Verification items for the finished model (mm, model axes). Face numbers are marked on the shaded views. Round coordinates to 2 decimals unless told otherwise and drop trailing zeros. Order: outer loops, then holes, each group sorted by start corner. A loop starts at its lowest first (then second) coordinate and runs counter-clockwise, first axis right, second up. Notation, with made-up numbers: (-21.75, 80) -> (19.25, 80) arc R29 ccw to (19.25, 116) -> close; hole circle Ø5 at (-14, 15). An arc over 180 degrees is marked (long way). Return JSON: item names as keys, results as strings. Group by question number.
Item 1: Scan lines: probe 1 along Z at (x, y) = (-12, 18.5); probe 2 along X at (y, z) = (26.5, 0); probe 3 along Z at (x, y) = (6, 37). Record each from-to range of solid material in increasing order. Write a range as from..to.
Item 2: Sectioned sample at D-D on x = 15. Record the cut outline in (y, z).
Item 3: Sectioned sample at C-C on z = 0. Record the cut outline in (x, y), plus the area to 3 significant figures.
Item 4: Draft check along X on the marked faces 1, 2 and 3. Enter one of: pulls with the +X half, pulls with the -X half, needs draft (parallel to the pull), parting line crosses it, or undercut.
Item 5: Sectioned sample at B-B on y = 18.5. Record the cut outline in (x, z).
Item 6: Sectioned sample at A-A on x = -14. Record the cut outline in (y, z), plus the area to 3 significant figures.
Autodesk Inventor part; units mm, degrees
ref_plane "YZ Plane" through (0, 0, 0) normal (1, 0, 0) x (0, 1, 0)
ref_plane "XZ Plane" through (0, 0, 0) normal (0, 1, 0) x (-1, 0, 0)
ref_plane "XY Plane" through (0, 0, 0) normal (0, 0, 1) x (1, 0, 0)
sketch "스케치1" plane through (0, 0, 0) normal (0, 1, 0) x (-1, 0, 0)
  line L0 (0, -16.483) -> (0, 16.483)
  line L1 (31.8385, 0) -> (-30.0309, 0)
  arc A0 (16.9497, 4.9497) -> (16.9497, -4.9497) centre (12, 0) ccw
  line L2 (12, -11) -> (0, -11)
  line L3 (12, 11) -> (0, 11)
  line L4 (12, 0) -> (19.7782, -7.7782)
  line L5 (12, 0) -> (23, 0) construction
  arc A1 (19.7782, -7.7782) -> (16.9497, -4.9497) centre (18.364, -6.364) ccw
  arc A2 (16.9497, 4.9497) -> (19.7782, 7.7782) centre (18.364, 6.364) ccw
  arc A3 (12, -11) -> (19.7782, -7.7782) centre (12, 0) ccw
  arc A4 (19.7782, 7.7782) -> (12, 11) centre (12, 0) ccw
  arc A5 (-16.9497, -4.9497) -> (-16.9497, 4.9497) centre (-12, 0) ccw
  line L6 (-12, -11) -> (0, -11)
  arc A6 (-16.9497, -4.9497) -> (-19.7782, -7.7782) centre (-18.364, -6.364) ccw
  arc A7 (-19.7782, 7.7782) -> (-16.9497, 4.9497) centre (-18.364, 6.364) ccw
  arc A8 (-19.7782, -7.7782) -> (-12, -11) centre (-12, 0) ccw
  arc A9 (-12, 11) -> (-19.7782, 7.7782) centre (-12, 0) ccw
  line L7 (-12, 11) -> (0, 11)
  point P0 (0, 0)
  dimension "d0" = 14
  dimension "d1" = 12
  dimension "d3" = 45
  dimension "d4" = 11
extrude "돌출1" add sketch "스케치1" along normal blind 50 contours L6 A8 A6 A5 L1 L0 | L0 L1 A0 L4 A3 L2 | L1 A5 A7 A9 L7 L0 | L0 L3 A4 A2 A0 L1 | L4 A1
properties part number "카메라 고정 중단"
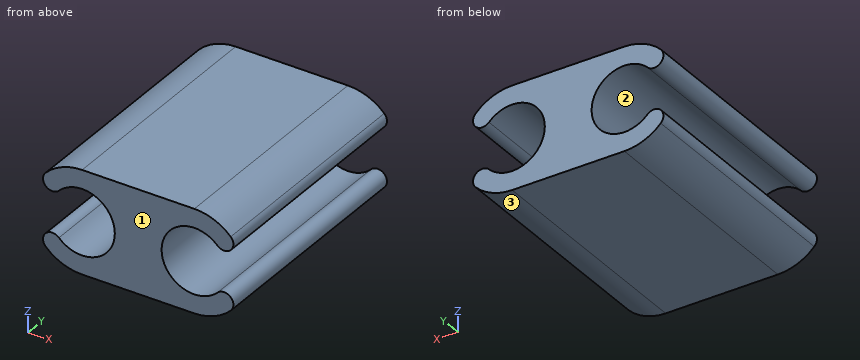
Recorded:
{
 "1": {"probe 1": "-11..-7, 7..11", "probe 2": "-5..5", "probe 3": "-11..-3.61, 3.61..11"},
 "2": {"outline": "(0, -10.58) -> (50, -10.58) -> (50, -6.32) -> (0, -6.32) -> close; (0, 6.32) -> (50, 6.32) -> (50, 10.58) -> (0, 10.58) -> close"},
 "3": {"outline": "(-5, 0) -> (5, 0) -> (5, 50) -> (-5, 50) -> close", "area": "500 mm²"},
 "4": {"face 1": "needs draft", "face 2": "undercut", "face 3": "pulls with the +X half"},
 "5": {"outline": "(-19.78, -7.78) arc R11 ccw to (-12, -11) -> (12, -11) arc R11 ccw to (19.78, -7.78) arc R2 ccw to (16.95, -4.95) arc R7 cw (long way) to (16.95, 4.95) arc R2 ccw to (19.78, 7.78) arc R11 ccw to (12, 11) -> (-12, 11) arc R11 ccw to (-19.78, 7.78) arc R2 ccw to (-16.95, 4.95) arc R7 cw (long way) to (-16.95, -4.95) arc R2 ccw to start"},
 "6": {"outline": "(0, -10.82) -> (50, -10.82) -> (50, -6.71) -> (0, -6.71) -> close; (0, 6.71) -> (50, 6.71) -> (50, 10.82) -> (0, 10.82) -> close", "area": "411 mm²"}
}
